from build123d import *

# Parameters (mm, degrees)
SKETCH2_R           = 1.25
SKETCH2_R_2         = 0.75
BOSS_EXTRUDE1_DEPTH = 0.5
CUT_EXTRUDE1_START  = -0.5
SKETCH3_R           = 0.75
CUT_EXTRUDE1_DEPTH  = 0.5
FILLET4_R           = 0.2
SKETCH4_R           = 0.375
BOSS_EXTRUDE2_DEPTH = 0.5
CUT_EXTRUDE3_DEPTH  = 8.133041914


with BuildPart() as part:
    # Sketch1 → Revolve1 (revolve)
    with BuildSketch(Plane(origin=(0, 0, 0), x_dir=(1, 0, 0), z_dir=(0, 1, 0)), mode=Mode.PRIVATE) as revolve1_sk:
        with BuildLine():
            Line((0, 0), (2.5, 0))
            ThreePointArc((2.5, 0), (3.207106781, -0.292893219), (3.5, -1))
            Line((3.5, -1), (3.5, -2.5))
            Line((3.5, -2.5), (3.25, -2.5))
            Line((3.25, -2.5), (3.25, -1))
            ThreePointArc((3.25, -1), (3.030330086, -0.469669914), (2.5, -0.25))
            Line((2.5, -0.25), (0, -0.25))
            Line((0, -0.25), (0, 0))
        make_face()
    revolve(revolve1_sk.sketch.rotate(Axis((0, 0, -4.115506763), (0, 0, 1)), 180), axis=Axis((0, 0, -4.115506763), (0, 0, 1)))

    # Sketch2 → Boss-Extrude1 (add)
    with BuildSketch(Plane(origin=(0, 0, 0), x_dir=(-1, 0, 0), z_dir=(0, 0, -1))):
        with Locations(Location((0, 0, 0), (0, 0, 180))):
            Circle(SKETCH2_R)
        Circle(SKETCH2_R_2, mode=Mode.SUBTRACT)
    extrude(amount=BOSS_EXTRUDE1_DEPTH)

    # Sketch3 → Cut-Extrude1 (cut)
    with BuildSketch(Plane(origin=(0, 0, 0), x_dir=(-1, 0, 0), z_dir=(0, 0, -1)).offset(CUT_EXTRUDE1_START)):
        Circle(SKETCH3_R)
    extrude(amount=CUT_EXTRUDE1_DEPTH, mode=Mode.SUBTRACT)

    # Fillet4
    fillet4_edges = [part.edges().sort_by_distance(p)[0] for p in [
        (-1.25, 0, -0.5),
    ]]
    fillet(fillet4_edges, radius=FILLET4_R)

    # Sketch4 → Boss-Extrude2 (add)
    # profile 1 of 3: a face of its own
    with BuildSketch(Plane.XY.offset(2.5)):
        with BuildLine():
            Line((0.75, 4.25), (0.75, 3.418698583))
            ThreePointArc((0.75, 3.418698583), (0, 3.5), (-0.75, 3.418698583))
            Line((-0.75, 3.418698583), (-0.75, 4.25))
            ThreePointArc((-0.75, 4.25), (0, 5), (0.75, 4.25))
        make_face()
        with Locations((0, 4.25)):
            Circle(SKETCH4_R, mode=Mode.SUBTRACT)
    # profile 2 of 3: a face of its own
    with BuildSketch(Plane.XY.offset(2.5)):
        with BuildLine():
            Line((3.305607966, -2.774519053), (2.585679821, -2.358868344))
            ThreePointArc((2.585679821, -2.358868344), (3.031088913, -1.75), (3.335679821, -1.059830239))
            Line((3.335679821, -1.059830239), (4.055607966, -1.475480947))
            ThreePointArc((4.055607966, -1.475480947), (4.330127019, -2.5), (3.305607966, -2.774519053))
        make_face()
        with Locations((3.680607966, -2.125)):
            Circle(SKETCH4_R, mode=Mode.SUBTRACT)
    # profile 3 of 3: a face of its own
    with BuildSketch(Plane.XY.offset(2.5)):
        with BuildLine():
            Line((-4.055607966, -1.475480947), (-3.335679821, -1.059830239))
            ThreePointArc((-3.335679821, -1.059830239), (-3.031088913, -1.75), (-2.585679821, -2.358868344))
            Line((-2.585679821, -2.358868344), (-3.305607966, -2.774519053))
            ThreePointArc((-3.305607966, -2.774519053), (-4.330127019, -2.5), (-4.055607966, -1.475480947))
        make_face()
        with Locations((-3.680607966, -2.125)):
            Circle(SKETCH4_R, mode=Mode.SUBTRACT)
    extrude(amount=-BOSS_EXTRUDE2_DEPTH)

    # Sketch5 → Cut-Extrude3 (cut, through all)
    with BuildSketch(Plane(origin=(0, 0, 0), x_dir=(-1, 0, 0), z_dir=(0, 0, -1))):
        with BuildLine():
            Line((-0.175, 2), (-0.175, -2))
            ThreePointArc((-0.175, -2), (0, -2.175), (0.175, -2))
            Line((0.175, -2), (0.175, 2))
            ThreePointArc((0.175, 2), (0, 2.175), (-0.175, 2))
        make_face()
        with BuildLine():
            Line((0.775, 2), (0.775, -2))
            ThreePointArc((0.775, -2), (0.6, -2.175), (0.425, -2))
            Line((0.425, -2), (0.425, 2))
            ThreePointArc((0.425, 2), (0.6, 2.175), (0.775, 2))
        make_face()
        with BuildLine():
            Line((1.375, 2), (1.375, -2))
            ThreePointArc((1.375, -2), (1.2, -2.175), (1.025, -2))
            Line((1.025, -2), (1.025, 2))
            ThreePointArc((1.025, 2), (1.2, 2.175), (1.375, 2))
        make_face()
        with BuildLine():
            Line((1.975, 2), (1.975, -2))
            ThreePointArc((1.975, -2), (1.8, -2.175), (1.625, -2))
            Line((1.625, -2), (1.625, 2))
            ThreePointArc((1.625, 2), (1.8, 2.175), (1.975, 2))
        make_face()
        with BuildLine():
            Line((-0.425, 2), (-0.425, -2))
            ThreePointArc((-0.425, -2), (-0.6, -2.175), (-0.775, -2))
            Line((-0.775, -2), (-0.775, 2))
            ThreePointArc((-0.775, 2), (-0.6, 2.175), (-0.425, 2))
        make_face()
        with BuildLine():
            Line((-1.025, 2), (-1.025, -2))
            ThreePointArc((-1.025, -2), (-1.2, -2.175), (-1.375, -2))
            Line((-1.375, -2), (-1.375, 2))
            ThreePointArc((-1.375, 2), (-1.2, 2.175), (-1.025, 2))
        make_face()
        with BuildLine():
            Line((-1.625, 2), (-1.625, -2))
            ThreePointArc((-1.625, -2), (-1.8, -2.175), (-1.975, -2))
            Line((-1.975, -2), (-1.975, 2))
            ThreePointArc((-1.975, 2), (-1.8, 2.175), (-1.625, 2))
        make_face()
    extrude(amount=-CUT_EXTRUDE3_DEPTH, mode=Mode.SUBTRACT)


solid = part.part
CAD build for the part. Positions are in the model's coordinates, mm. A direction names the side the tool comes from. Give positions to 0.01 mm unless a question says otherwise; leave off trailing zeros. Write each loop counter-clockwise with the first axis right and the second up, starting at its lowest first coordinate (ties: lowest second). Pieces come first, ordered by that corner, then holes. Notation, with made-up numbers: (51.5, 8.5) - (63.5, 8.5) arc R5 ccw to (63.5, 15.5) - close; hole circle Ø3 at (-26.75, 52). An arc over 180 degrees is marked (long way). Put each result on its own line as item: value.
(1) Saw through at A-A (x = 0). Count the separate pieces of the cut face and the enclosed holes in it, then the cut area to 3 significant figures.
Working result:
separate pieces: 5
enclosed holes: 0
area: 2.46 mm^2
(2) Saw through at D-D (z = 0.65). List the corners of the cut face in (x, y).
Working result:
outline: circle Ø6.87 at (0, 0); hole circle Ø6.33 at (0, 0)
(3) Saw through at C-C (z = 1.35). List the corners of the cut face in (x, y).
Working result:
outline: circle Ø7 at (0, 0); hole circle Ø6.5 at (0, 0)
(4) Drop flat-ended pins along their axis: pin 1 Ø5 at (x, y) = (2, 1) entering from -Z; pin 2 Ø2 at (x, y) = (4, -2.5) entering from -Z; pin 3 Ø1 at (y, z) = (1, 1) entering from +X. Give the stop position or say it passes through.
Working result:
pin 1: z = -0.5
pin 2: z = 2
pin 3: x = 3.46
(5) Tool access for faces 1 (the flat face through (3.1, -2.2, 2)), 2 (the cylindrical face through (-1.25, -0.05, -0.15)), 3 (the flat face through (-3.29, -1.75, 2)), 4 (the cylindrical face through (2.579, 1.978, 1.74)), 5 (the cylindrical face through (-0.715, 0.225, -0.203)): list every direction of +Z, -Z, +X, -X, +Y, -Y with a clear straight run to the whole face (end or side of a thin tool).
Working result:
face 1: -Z, +X, -Y
face 2: -Z
face 3: -Z, -X, -Y
face 4: +Z
face 5: +Z, -Z
(6) Wall check: L1, parallel to Y at x = 0, z = 2.1 (3 decimals); L2, parallel to Y at x = 0, z = -0.1; L3, parallel to X at y = 1.75, z = 2.05. Give the ranges that are in metal, low to high.
Working result:
L1: -3.5 to -3.25, 3.25 to 3.875, 4.625 to 5
L2: -1.25 to -0.75, 0.75 to 1.25
L3: -3.03 to -2.74, 2.74 to 3.03
